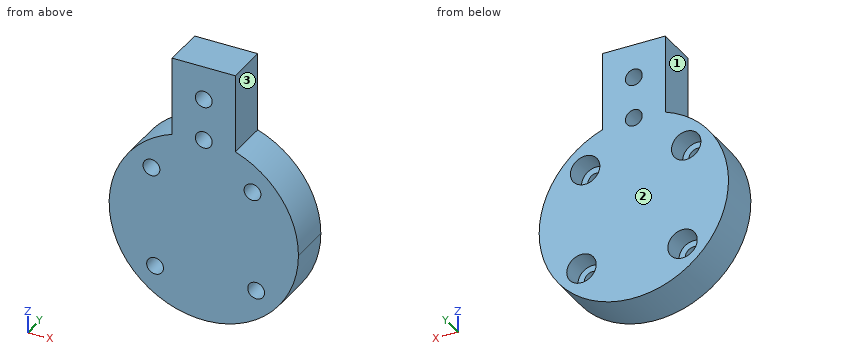
```python
from build123d import *

# Parameters (mm, degrees)
BOSS_EXTRUDE1_DEPTH = 10
SKETCH2_R           = 2
CUT_EXTRUDE1_DEPTH  = 10
SKETCH3_R           = 2
CUT_EXTRUDE2_DEPTH  = 10
SKETCH4_R           = 3.5
CUT_EXTRUDE3_DEPTH  = 5


with BuildPart() as part:
    # Sketch1 → Boss-Extrude1 (new body)
    with BuildSketch(Plane(origin=(0, 0, 0), x_dir=(1, 0, 0), z_dir=(0, 1, 0))):
        with BuildLine():
            ThreePointArc((7.5, -21.213203436), (0, -22.5), (-7.5, -21.213203436))
            Line((-7.5, -21.213203436), (-7.5, -40))
            Line((-7.5, -40), (7.5, -40))
            Line((7.5, -40), (7.5, -21.213203436))
        make_face()
        with BuildLine():
            Line((-7.5, -21.213203436), (-7.5, 0))
            Line((-7.5, 0), (7.5, 0))
            Line((7.5, 0), (7.5, -21.213203436))
            ThreePointArc((7.5, -21.213203436), (18.371173071, -12.990381057), (22.5, 0))
            ThreePointArc((22.5, 0), (-12.990381057, 18.371173071), (-7.5, -21.213203436))
        make_face()
        with BuildLine():
            Line((7.5, 0), (-7.5, 0))
            Line((-7.5, 0), (-7.5, -21.213203436))
            ThreePointArc((-7.5, -21.213203436), (0, -22.5), (7.5, -21.213203436))
            Line((7.5, -21.213203436), (7.5, 0))
        make_face()
    extrude(amount=BOSS_EXTRUDE1_DEPTH)

    # Sketch2 → Cut-Extrude1 (cut)
    with BuildSketch(Plane(origin=(0, 10, 0), x_dir=(1, 0, 0), z_dir=(0, 1, 0))):
        with Locations((-11.579332818, 12.446648203)):
            Circle(SKETCH2_R)
        with Locations((12.446648203, 11.579332818)):
            Circle(SKETCH2_R)
        with Locations((11.579332818, -12.446648203)):
            Circle(SKETCH2_R)
        with Locations((-12.446648203, -11.579332818)):
            Circle(SKETCH2_R)
    extrude(amount=-CUT_EXTRUDE1_DEPTH, mode=Mode.SUBTRACT)

    # Sketch3 → Cut-Extrude2 (cut)
    with BuildSketch(Plane(origin=(0, 10, 0), x_dir=(1, 0, 0), z_dir=(0, 1, 0))):
        with Locations((0, -22)):
            Circle(SKETCH3_R)
        with Locations((0, -32)):
            Circle(SKETCH3_R)
    extrude(amount=-CUT_EXTRUDE2_DEPTH, mode=Mode.SUBTRACT)

    # Sketch4 → Cut-Extrude3 (cut)
    with BuildSketch(Plane(origin=(0, 10, 0), x_dir=(1, 0, 0), z_dir=(0, 1, 0))):
        with Locations((-11.579332818, 12.446648203)):
            Circle(SKETCH4_R)
        with Locations((12.446648203, 11.579332818)):
            Circle(SKETCH4_R)
        with Locations((11.579332818, -12.446648203)):
            Circle(SKETCH4_R)
        with Locations((-12.446648203, -11.579332818)):
            Circle(SKETCH4_R)
    extrude(amount=-CUT_EXTRUDE3_DEPTH, mode=Mode.SUBTRACT)


solid = part.part
```
Source: CAD feature listing. Evaluate the final solid. Frame: model axes, mm. Face numbers are marked on the shaded views. A direction names the side the tool comes from. Give positions to 0.01 mm unless a question says otherwise; leave off trailing zeros. Order: outer loops, then holes, each group sorted by start corner. A loop starts at its lowest first (then second) coordinate and runs counter-clockwise, first axis right, second up.
(1) Section query A-A (x = 0). Return the cut outline in (y, z), plus the area to 3 significant figures.
(2) Access query for the marked faces 1, 2 and 3. Directions: +Z, -Z, +X, -X, +Y, -Y. A direction counts if a zero-diameter tool reaches every point of the face in a straight line with its end or side. Return the directions, or none.
(3) Section query B-B (z = 22). Return the cut outline in (x, y), plus the area to 3 significant figures.
(4) Section query D-D (y = 1.5). Return the cut outline in (x, z), plus the area to 3 significant figures.
(5) Section query C-C (y = 6.75). Return the cut outline in (x, z), plus the area to 3 significant figures.
(6) Contact query for flat-ended pins moving along their axis: P1, Ø4.5, axis at x = 0, z = 32, coming from the +Y side; P2, Ø5, axis at y = 4, z = 30.5, coming from the -X side; P3, Ø2, axis at x = -14, z = 11.5, coming from the +Y side; P4, Ø1.5, axis at x = -12, y = 8.5, coming from the -Z side. Output: stop coordinate, or through.
(7) Material intervals for line 1 along Z through (x, y) = (-12, 6.75); line 2 along Z through (x, y) = (-1.5, 1.5); line 3 along X through (y, z) = (3.75, 37), sorted ascending.
Outcome:
1. outline: (0, -22.5) - (10, -22.5) - (10, 20) - (0, 20) - close; (0, 24) - (10, 24) - (10, 30) - (0, 30) - close; (0, 34) - (10, 34) - (10, 40) - (0, 40) - close
1. area: 545 mm2
2. face 1: +Z, -X, +Y, -Y
2. face 2: +Z, -Z, +X, -X, +Y
2. face 3: +Z, +X, +Y, -Y
3. outline: (-7.5, 0) - (-2, 0) - (-2, 10) - (-7.5, 10) - close; (2, 0) - (7.5, 0) - (7.5, 10) - (2, 10) - close
3. area: 110 mm2
4. outline: (-7.5, 21.21) arc R22.5 ccw (long way) to (7.5, 21.21) - (7.5, 40) - (-7.5, 40) - close; hole circle Ø4 at (-12.45, 11.58); hole circle Ø4 at (-11.58, -12.45); hole circle Ø4 at (0, 22); hole circle Ø4 at (0, 32); hole circle Ø4 at (11.58, 12.45); hole circle Ø4 at (12.45, -11.58)
4. area: 1,780 mm2
5. outline: (-7.5, 21.21) arc R22.5 ccw (long way) to (7.5, 21.21) - (7.5, 40) - (-7.5, 40) - close; hole circle Ø7 at (-12.45, 11.58); hole circle Ø7 at (-11.58, -12.45); hole circle Ø4 at (0, 22); hole circle Ø4 at (0, 32); hole circle Ø7 at (11.58, 12.45); hole circle Ø7 at (12.45, -11.58)
5. area: 1,680 mm2
6. P1: stops at y = 10
6. P2: stops at x = -7.5
6. P3: stops at y = 5
6. P4: stops at z = -19.49
7. line 1: z = -19.03 to -15.92, -8.97 to 8.11, 15.05 to 19.03
7. line 2: z = -22.45 to 20.68, 23.32 to 30.68, 33.32 to 40
7. line 3: x = -7.5 to 7.5
